Build history of the part. All positions in model axes, mm. A direction names the side the tool comes from. Coordinates: 2 decimals unless noted, no trailing zeros. Loops run counter-clockwise (first coordinate to the right, second up) from the corner with the lowest first, then second, coordinate; pieces in that order, holes last.
Item 1: Cut at C-C (z = -12). List the corners of the cut face in (x, y).
Item 2: Drill centre lines: line 1 along Y through (x, z) = (2, -10.5); line 2 along Z through (x, y) = (8.5, 8.25); line 3 along Z through (x, y) = (8, -1.5). Where is each one in solid material? Low to high.
Item 3: Flat gauge pins, fed straight in: pin 1 (2 mm diameter, centred on y = 5, z = -12, fed in from -X); pin 2 (0.9 mm diameter, centred on x = -1.5, z = -12, fed in from -Y). Where does each tip first touch, or does it go through?
Item 4: 3-axis set-ups, long thin cutter, end or side, ignore diameter. For faces 1 (the face through (8.242, -0.382, -19.839)), 2 (the face through (-1, 2.718, -13)), 3 (the face through (0, 0, 0)), 4 (the face through (11.68, 6.38, -12.89)), 5 (the face through (-1, 9.601, -13)): which of +Z, -Z, +X, -X, +Y, -Y reach the whole face in a straight line?
Item 5: Mould opens along Z. For faces 6 (the face through (0, 6, 10.871)), 7 (the face through (-11.684, 6, 0)), 8 (the face through (6, -1, -19.025)) say: released by +Z, released by -Z, zero draft, split by the parting line, or undercut.
Item 6: Cut at B-B (y = 4). List the corners of the cut face in (x, z), and give its area (3 significant figures).
Item 7: Cut at D-D (y = 10). List the corners of the cut face in (x, z), and give its area (3 significant figures).
Item 8: Cut at A-A (x = -2). List the corners of the cut face in (y, z), and give its area (3 significant figures).
from build123d import *

# Parameters (mm, degrees)
SKETCH1_W           = 23.368
SKETCH1_H           = 21.7424
BOSS_EXTRUDE1_DEPTH = 12.319
BOSS_EXTRUDE2_DEPTH = 4.0894
SKETCH3_R           = 3.4163
BOSS_EXTRUDE3_DEPTH = 4.064
BOSS_EXTRUDE4_DEPTH = 1.651
CUT_EXTRUDE1_START  = -1.651
SKETCH5_R           = 0.381
CUT_EXTRUDE1_DEPTH  = 1.651


with BuildPart() as part:
    # Sketch1 → Boss-Extrude1 (new body)
    with BuildSketch(Plane(origin=(0, 0, 0), x_dir=(1, 0, 0), z_dir=(0, 1, 0))):
        Rectangle(SKETCH1_W, SKETCH1_H)
    extrude(amount=BOSS_EXTRUDE1_DEPTH)

    # Sketch2 → Boss-Extrude2 (add)
    with BuildSketch(Plane(origin=(0, 0, -10.8712), x_dir=(-1, 0, 0), z_dir=(0, 0, -1))):
        with BuildLine():
            Line((-0.416257508, 2.7178), (2.6162, 2.7178))
            Line((2.6162, 2.7178), (2.6162, 9.6012))
            Line((2.6162, 9.6012), (-0.416257508, 9.6012))
            ThreePointArc((-0.416257508, 9.6012), (-11.684, 6.1595), (-0.416257508, 2.7178))
        make_face()
    extrude(amount=BOSS_EXTRUDE2_DEPTH)

    # Sketch3 → Boss-Extrude3 (add)
    with BuildSketch(Plane(origin=(0, 0, -14.9606), x_dir=(-1, 0, 0), z_dir=(0, 0, -1))):
        with Locations((-5.5245, 6.1595)):
            Circle(SKETCH3_R)
    extrude(amount=BOSS_EXTRUDE3_DEPTH)

    # Sketch4 → Boss-Extrude4 (add)
    with BuildSketch(Plane(origin=(0, 0, -19.0246), x_dir=(-1, 0, 0), z_dir=(0, 0, -1))):
        with BuildLine():
            Line((-8.920321777, 5.786002808), (-7.544319644, -6.724554463))
            ThreePointArc((-7.544319644, -6.724554463), (-5.5245, -8.5344), (-3.504680356, -6.724554463))
            Line((-3.504680356, -6.724554463), (-2.128678223, 5.786002808))
            ThreePointArc((-2.128678223, 5.786002808), (-5.5245, 9.5758), (-8.920321777, 5.786002808))
        make_face()
    extrude(amount=BOSS_EXTRUDE4_DEPTH)

    # Sketch5 → Cut-Extrude1 (cut)
    with BuildSketch(Plane(origin=(0, 0, -20.6756), x_dir=(-1, 0, 0), z_dir=(0, 0, -1)).offset(CUT_EXTRUDE1_START)):
        with Locations((-5.5245, -6.5024)):
            Circle(SKETCH5_R)
        with Locations((-5.5245, -4.4704)):
            Circle(SKETCH5_R)
        with Locations((-5.5245, -2.4384)):
            Circle(SKETCH5_R)
        with Locations((-5.5245, -0.4064)):
            Circle(SKETCH5_R)
        with Locations((-5.5245, 1.6256)):
            Circle(SKETCH5_R)
    extrude(amount=CUT_EXTRUDE1_DEPTH, mode=Mode.SUBTRACT)


solid = part.part
Filled sheet:
1. outline: (-2.62, 2.72) - (0.42, 2.72) arc R6.16 ccw (long way) to (0.42, 9.6) - (-2.62, 9.6) - close
2. line 1: y = 0 to 12.32
2. line 2: z = -14.96 to 10.87
2. line 3: z = -20.68 to -19.02
3. pin 1: stops at x = -2.62
3. pin 2: stops at y = 2.72
4. face 1: -Z, +X, -Y
4. face 2: -Z, -X, -Y
4. face 3: +Z, +X, -X, -Y
4. face 4: none
4. face 5: -Z, -X, +Y
5. face 6: released by +Z
5. face 7: zero draft
5. face 8: undercut
6. outline: (-11.68, -10.87) - (-2.62, -10.87) - (-2.62, -14.96) - (2.88, -14.96) - (2.88, -19.02) - (2.33, -19.02) - (2.33, -20.68) - (8.72, -20.68) - (8.72, -19.02) - (8.17, -19.02) - (8.17, -14.96) - (11.29, -14.96) - (11.29, -10.87) - (11.68, -10.87) - (11.68, 10.87) - (-11.68, 10.87) - close
6. area: 597 mm2
7. outline: (-11.68, -10.87) - (0.71, -10.87) - (0.71, -14.96) - (10.34, -14.96) - (10.34, -10.87) - (11.68, -10.87) - (11.68, 10.87) - (-11.68, 10.87) - close
7. area: 547 mm2
8. outline: (0, -10.87) - (2.72, -10.87) - (2.72, -14.96) - (9.6, -14.96) - (9.6, -10.87) - (12.32, -10.87) - (12.32, 10.87) - (0, 10.87) - close
8. area: 296 mm2
